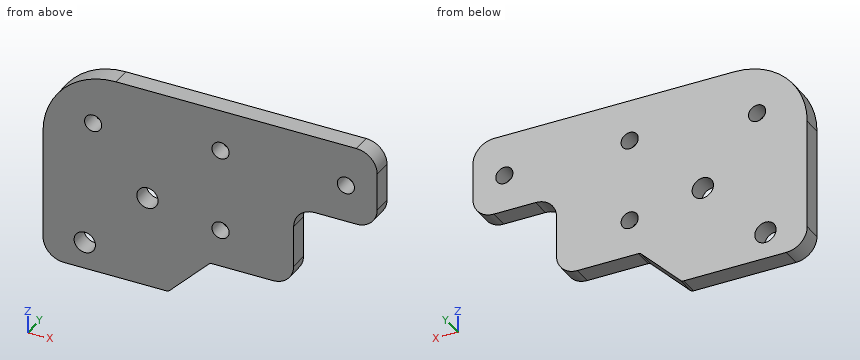
from build123d import *

# Parameters (mm, degrees)
SKETCH1_R           = 2.05
BOSS_EXTRUDE1_DEPTH = 4.5
SKETCH2_R           = 2.55
SKETCH2_R_2         = 2.05
CUT_EXTRUDE1_DEPTH  = 94.921509783
FILLET1_R           = 5
FILLET2_R           = 17.5
FILLET3_R           = 1


with BuildPart() as part:
    # Sketch1 → Boss-Extrude1 (new body)
    with BuildSketch(Plane(origin=(0, 0, 0), x_dir=(1, 0, 0), z_dir=(0, 1, 0))):
        Polygon((80, 19), (60, 19), (60, 39), (40, 39), (30, 49), (0, 49), (0, 0), (80, 0), align=None)
        with Locations(Location((72.5, 10, 0), (0, 0, 270))):
            Circle(SKETCH1_R, mode=Mode.SUBTRACT)
        with Locations(Location((42.5, 10, 0), (0, 0, 270))):
            Circle(SKETCH1_R, mode=Mode.SUBTRACT)
        with Locations(Location((42.5, 30, 0), (0, 0, 270))):
            Circle(SKETCH1_R, mode=Mode.SUBTRACT)
    extrude(amount=BOSS_EXTRUDE1_DEPTH)

    # Sketch2 → Cut-Extrude1 (cut, through all)
    with BuildSketch(Plane(origin=(0, 4.5, 0), x_dir=(1, 0, 0), z_dir=(0, 1, 0))):
        with Locations(Location((25, 27, 0), (0, 0, 270))):
            Circle(SKETCH2_R)
        with Locations(Location((10, 42.5, 0), (0, 0, 270))):
            Circle(SKETCH2_R)
        with Locations(Location((12, 12, 0), (0, 0, 270))):
            Circle(SKETCH2_R_2)
    extrude(amount=-CUT_EXTRUDE1_DEPTH, mode=Mode.SUBTRACT)

    # Fillet1
    fillet1_edges = [part.edges().sort_by_distance(p)[0] for p in [
        (0, 2.25, -49),
        (60, 2.25, -39),
        (60, 2.25, -19),
        (80, 2.25, -19),
        (80, 2.25, 0),
    ]]
    fillet(fillet1_edges, radius=FILLET1_R)

    # Fillet2
    fillet2_edges = [part.edges().sort_by_distance(p)[0] for p in [
        (0, 2.25, 0),
    ]]
    fillet(fillet2_edges, radius=FILLET2_R)

    # Fillet3
    fillet3_edges = [part.edges().sort_by_distance(p)[0] for p in [
        (30, 2.25, -49),
        (40, 2.25, -39),
    ]]
    fillet(fillet3_edges, radius=FILLET3_R)


solid = part.part
CAD build for the part. Positions are in the model's coordinates, mm. Give positions to 0.01 mm unless a question says otherwise; leave off trailing zeros. Order: outer loops, then holes, each group sorted by start corner. A loop starts at its lowest first (then second) coordinate and runs counter-clockwise, first axis right, second up. Notation, with made-up numbers: (81.25, -39) -> (104.25, -39) arc R21 cw to (104.25, -21) -> close; hole circle Ø8 at (77, 61). An arc over 180 degrees is marked (long way). Return JSON: item names as keys, results as strings.
Q1. Drill centre lines: line 1 (X direction, y = 3.5, z = -27); line 2 (Z direction, x = 11.5, y = 0.9); line 3 (X direction, y = 2.75, z = -30). Where is each one in solid material? Low to high.
Working result:
{"line 1": "0 to 22.45, 27.55 to 60", "line 2": "-49 to -44.56, -40.44 to -13.99, -10.01 to -1.06", "line 3": "0 to 40.45, 44.55 to 60"}
Q2. Saw through at C-C (y = 0.75). Write the cut outline in (x, z).
Working result:
{"outline": "(0, -44) arc R5 ccw to (5, -49) -> (29.59, -49) arc R1 ccw to (30.29, -48.71) -> (39.71, -39.29) arc R1 cw to (40.41, -39) -> (55, -39) arc R5 ccw to (60, -34) -> (60, -24) arc R5 cw to (65, -19) -> (75, -19) arc R5 ccw to (80, -14) -> (80, -5) arc R5 ccw to (75, 0) -> (17.5, 0) arc R17.5 ccw to (0, -17.5) -> close; hole circle Ø5.1 at (10, -42.5); hole circle Ø4.1 at (12, -12); hole circle Ø5.1 at (25, -27); hole circle Ø4.1 at (42.5, -30); hole circle Ø4.1 at (42.5, -10); hole circle Ø4.1 at (72.5, -10)"}
Q3. Flat gauge pins, fed straight in: pin 1 (1.5 mm diameter, centred on y = 2.5, z = -34.5, fed in from +X); pin 2 (1 mm diameter, centred on x = 48, y = 1, fed in from -Z); pin 3 (3 mm diameter, centred on x = 10, z = -42.5, fed in from -Y). Where does each tip first touch, or does it go through?
Working result:
{"pin 1": "x = 60", "pin 2": "z = -39", "pin 3": "through"}
Q4. Saw through at A-A (x = 42.5). Write the cut outline in (y, z), then the cut area to 3 significant figures.
Working result:
{"outline": "(0, -39) -> (4.5, -39) -> (4.5, -32.05) -> (0, -32.05) -> close; (0, -27.95) -> (4.5, -27.95) -> (4.5, -12.05) -> (0, -12.05) -> close; (0, -7.95) -> (4.5, -7.95) -> (4.5, 0) -> (0, 0) -> close", "area": "139 mm²"}
Q5. Saw through at B-B (z = -42.5). Write the cut outline in (x, y), then the cut area to 3 significant figures.
Working result:
{"outline": "(0, 0) -> (7.45, 0) -> (7.45, 4.5) -> (0, 4.5) -> close; (12.55, 0) -> (36.5, 0) -> (36.5, 4.5) -> (12.55, 4.5) -> close", "area": "141 mm²"}
Q6. Saw through at D-D (x = 72.5). Write the cut outline in (y, z), then the cut area to 4 significant figures.
Working result:
{"outline": "(0, -19) -> (4.5, -19) -> (4.5, -12.05) -> (0, -12.05) -> close; (0, -7.95) -> (4.5, -7.95) -> (4.5, 0) -> (0, 0) -> close", "area": "67.05 mm²"}
